from build123d import *

# Parameters (mm, degrees)
SKETCH_1_R               = 12.25
SKETCH_1_R_2             = 9.25
EXTRUDE_1_DEPTH          = 10
CUT_EXTRUDE_1_DEPTH      = 1
CUT_EXTRUDE_1_DEPTH_BACK = 11
SKETCH_3_W               = 9.638758803
SKETCH_3_H               = 7
CUT_EXTRUDE_2_DEPTH      = 11
SKETCH_4_R               = 1.65
CUT_EXTRUDE_3_DEPTH      = 24.478713764
FILLET_1_R               = 1


with BuildPart() as part:
    # ｽｹｯﾁ1 → ﾎﾞｽ - 押し出し1 (new body)
    with BuildSketch(Plane.XY):
        Circle(SKETCH_1_R)
        Circle(SKETCH_1_R_2, mode=Mode.SUBTRACT)
    extrude(amount=EXTRUDE_1_DEPTH)

    # ｽｹｯﾁ2 → ｶｯﾄ - 押し出し1 (cut, two sides)
    with BuildSketch(Plane.XY.offset(10)) as cut_extrude_1_sk:
        with BuildLine():
            Line((-5.177073706, 11.102270391), (-3.909218921, 8.38334703))
            ThreePointArc((-3.909218921, 8.38334703), (0, 9.25), (3.909218921, 8.38334703))
            Line((3.909218921, 8.38334703), (5.177073706, 11.102270391))
            ThreePointArc((5.177073706, 11.102270391), (0, 12.25), (-5.177073706, 11.102270391))
        make_face()
    extrude(amount=CUT_EXTRUDE_1_DEPTH, mode=Mode.SUBTRACT)
    extrude(cut_extrude_1_sk.sketch, amount=-CUT_EXTRUDE_1_DEPTH_BACK, mode=Mode.SUBTRACT)

    # ｽｹｯﾁ3 → ｶｯﾄ - 押し出し2 (cut, through all)
    with BuildSketch(Plane.XY.offset(10)):
        with Locations((-16.558736284, 0)):
            Rectangle(SKETCH_3_W, SKETCH_3_H)
        with Locations((16.558736284, 0)):
            Rectangle(SKETCH_3_W, SKETCH_3_H)
    extrude(amount=-CUT_EXTRUDE_2_DEPTH, mode=Mode.SUBTRACT)

    # ｽｹｯﾁ4 → ｶｯﾄ - 押し出し3 (cut, through all)
    with BuildSketch(Plane(origin=(11.739356882, 0, 0), x_dir=(0, 0, -1), z_dir=(1, 0, 0))):
        with Locations((-5, 0)):
            Circle(SKETCH_4_R)
    extrude(amount=-CUT_EXTRUDE_3_DEPTH, mode=Mode.SUBTRACT)

    # ﾌｨﾚｯﾄ1
    fillet_1_edges = [part.edges().sort_by_distance(p)[0] for p in [
        (-5.177073706, 11.102270391, 5),
        (5.177073706, 11.102270391, 5),
    ]]
    fillet(fillet_1_edges, radius=FILLET_1_R)


solid = part.part
The listing builds one solid part. Answer for the finished solid, in the listing's coordinates (mm). A direction names the side the tool comes from. Give positions to 0.01 mm unless a question says otherwise; leave off trailing zeros. Write each loop counter-clockwise with the first axis right and the second up, starting at its lowest first coordinate (ties: lowest second). Pieces come first, ordered by that corner, then holes. Notation, with made-up numbers: (-27.75, -9.75) -> (-14.75, -9.75) arc R23 ccw to (-14.75, 12.25) -> close; hole circle Ø2 at (15, -13). An arc over 180 degrees is marked (long way). One line per question, with ' | ' between items. Start each with the question number.
1. Section C-C (x = -5.75) is taken. Determine the outline of the cut face in (y, z), plus the area to 3 significant figures.
2. For faces 4 (the flat face through (4.32, 9.26, 5.07)), 5 (the cylindrical face through (-0.35, -9.243, 4.93)), determine the directions among +Z, -Z, +X, -X, +Y, -Y from which every point of the face is accessible in a straight line to the end or side of a thin tool.
3. Section B-B (y = 0) is taken. Determine the outline of the cut face in (x, z), plus the area to 3 significant figures.
4. Section A-A (z = 5) is taken. Determine the outline of the cut face in (x, y).
5. For a pull along Z with two mould halves and no side action, classify faces 1 (the flat face through (11.739, -2, 6)), 2 (the flat face through (-4.4, -8.4, 0)), 3 (the cylindrical face through (-10.4, -1.6, 5.4)) as pulls with the +Z half, pulls with the -Z half, needs draft (parallel to the pull), parting line crosses it, or undercut.
6. Given pin 1 Ø12 at (x, y) = (2.5, 0.5) entering from -Z; pin 2 Ø5.5 at (y, z) = (0, 5) entering from +X; pin 3 Ø3 at (y, z) = (-7.5, 2.5) entering from +X; pin 4 Ø1 at (x, z) = (0.5, 8) entering from +Y, each flat-ended and moving along its own axis, determine where each tip first touches the part or whether it passes through.
7. Section D-D (y = 6.5) is taken. Determine the outline of the cut face in (x, z).
8. Find the intervals of material crossed by probe 1 along Z at (x, y) = (-10, 0); probe 2 along X at (y, z) = (-3.5, 6.75); probe 3 along Y at (x, z) = (6.5, 2.5), in increasing order.
Response values:
1) outline: (-10.82, 0) -> (-7.25, 0) -> (-7.25, 10) -> (-10.82, 10) -> close; (7.25, 0) -> (10.73, 0) -> (10.73, 10) -> (7.25, 10) -> close | area: 70.5 mm2
2) face 4: +Z, -Z, +Y | face 5: +Z, -Z
3) outline: (-11.74, 0) -> (-9.25, 0) -> (-9.25, 3.35) -> (-11.74, 3.35) -> close; (-11.74, 6.65) -> (-9.25, 6.65) -> (-9.25, 10) -> (-11.74, 10) -> close; (9.25, 0) -> (11.74, 0) -> (11.74, 3.35) -> (9.25, 3.35) -> close; (9.25, 6.65) -> (11.74, 6.65) -> (11.74, 10) -> (9.25, 10) -> close | area: 33.4 mm2
4) outline: (-11.74, -3.5) arc R12.25 ccw to (11.74, -3.5) -> (11.74, -1.65) -> (9.1, -1.65) arc R9.25 cw to (-9.1, -1.65) -> (-11.74, -1.65) -> close; (-11.74, 1.65) -> (-9.1, 1.65) arc R9.25 cw to (-3.91, 8.38) -> (-4.74, 10.16) arc R1 ccw to (-6.14, 10.6) arc R12.25 ccw to (-11.74, 3.5) -> close; (3.91, 8.38) arc R9.25 cw to (9.1, 1.65) -> (11.74, 1.65) -> (11.74, 3.5) arc R12.25 ccw to (6.14, 10.6) arc R1 ccw to (4.74, 10.16) -> close
5) face 1: needs draft | face 2: pulls with the -Z half | face 3: undercut
6) pin 1: through | pin 2: x = 11.74 | pin 3: x = 10.68 | pin 4: y = -9.2
7) outline: (-10.38, 0) -> (-6.58, 0) -> (-6.58, 10) -> (-10.38, 10) -> close; (6.58, 0) -> (10.38, 0) -> (10.38, 10) -> (6.58, 10) -> close
8) probe 1: 0 to 3.35, 6.65 to 10 | probe 2: -11.74 to -8.56, 8.56 to 11.74 | probe 3: -10.38 to -6.58, 6.58 to 10.38
